Here's how the part is built. I have some questions about the finished solid (model axes, mm). Face numbers are marked on the shaded views. A direction names the side the tool comes from. Give positions to 0.01 mm unless a question says otherwise; leave off trailing zeros. Write each loop counter-clockwise with the first axis right and the second up, starting at its lowest first coordinate (ties: lowest second). Pieces come first, ordered by that corner, then holes. Notation, with made-up numbers: (12.25, 40) -> (71.25, 40) arc R26 cw to (71.25, 59) -> close; hole circle Ø7 at (69.5, 86.25). An arc over 180 degrees is marked (long way). Use one line per item in the form item = value.
```python
from build123d import *

# Parameters (mm, degrees)
SALIENTE_EXTRUIR2_DEPTH      = 2.5
SALIENTE_EXTRUIR2_DEPTH_BACK = 2.5
CROQUIS2_R                   = 8
CROQUIS2_R_2                 = 2.5
REDONDEO1_R                  = 0.5
REDONDEO2_R                  = 0.1
CROQUIS3_R                   = 7
CROQUIS3_R_2                 = 4
CORTAR_EXTRUIR1_DEPTH        = 0.1
CORTAR_EXTRUIR2_START        = -0.1
CROQUIS4_R                   = 7
CROQUIS4_R_2                 = 4
CORTAR_EXTRUIR2_DEPTH        = 0.1


with BuildPart() as part:
    # Croquis2 → Saliente-Extruir2 (new, two sides: drawn at the far end of the back side and taken through both)
    with BuildSketch(Plane(origin=(0, 0, 0), x_dir=(0, 0, -1), z_dir=(1, 0, 0)).offset(-SALIENTE_EXTRUIR2_DEPTH_BACK)):
        Circle(CROQUIS2_R)
        Circle(CROQUIS2_R_2, mode=Mode.SUBTRACT)
    extrude(amount=SALIENTE_EXTRUIR2_DEPTH + SALIENTE_EXTRUIR2_DEPTH_BACK)

    # Redondeo1
    redondeo1_edges = [part.edges().sort_by_distance(p)[0] for p in [
        (-2.5, 0, 8),
        (2.5, 0, 8),
    ]]
    fillet(redondeo1_edges, radius=REDONDEO1_R)

    # Redondeo2
    redondeo2_edges = [part.edges().sort_by_distance(p)[0] for p in [
        (-2.5, 0, 2.5),
        (2.5, 0, 2.5),
    ]]
    fillet(redondeo2_edges, radius=REDONDEO2_R)

    # Croquis3 → Cortar-Extruir1 (cut)
    with BuildSketch(Plane.ZY.offset(2.5)):
        Circle(CROQUIS3_R)
        Circle(CROQUIS3_R_2, mode=Mode.SUBTRACT)
    extrude(amount=-CORTAR_EXTRUIR1_DEPTH, mode=Mode.SUBTRACT)

    # Croquis4 → Cortar-Extruir2 (cut)
    with BuildSketch(Plane(origin=(2.5, 0, 0), x_dir=(0, 0, -1), z_dir=(1, 0, 0)).offset(CORTAR_EXTRUIR2_START)):
        with Locations(Location((0, 0, 0), (0, 0, 180))):
            Circle(CROQUIS4_R)
        with Locations(Location((0, 0, 0), (0, 0, 180))):
            Circle(CROQUIS4_R_2, mode=Mode.SUBTRACT)
    extrude(amount=CORTAR_EXTRUIR2_DEPTH, mode=Mode.SUBTRACT)


solid = part.part
```
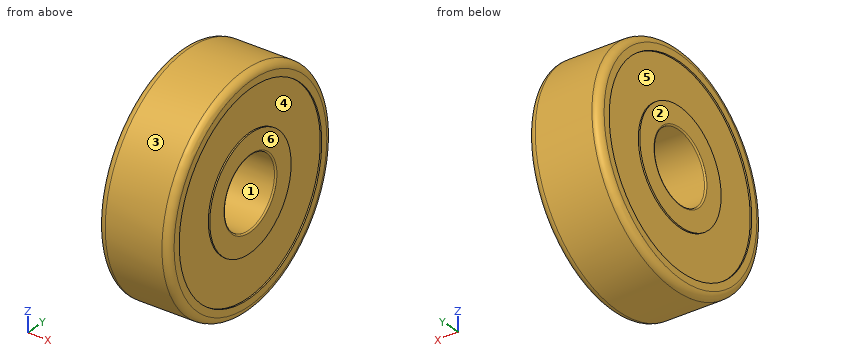
Q1. Will these pins go through, and if not, where does the flat tip stop? pin 1 Ø5 at (y, z) = (-1.5, -2) entering from -X; pin 2 Ø1 at (x, y) = (-2, 1) entering from +Z; pin 3 Ø1 at (y, z) = (-5.5, 0.5) entering from +X; pin 4 Ø1 at (x, z) = (1, 2.5) entering from +Y.
Result set:
pin_1 = -2.5
pin_2 = 7.98
pin_3 = 2.4
pin_4 = 7.75
Q2. Which directions (+Z, -Z, +X, -X, +Y, -Y) give clear straight access to the entire face, cutting with the end or side of a thin tool? Please do the marked faces 4, 5 and 6.
Result set:
face_4 = +X
face_5 = -X
face_6 = +Z, -Z, +X, +Y, -Y
Q3. If we mould it in two halves opening along Y, with no side actions, what happens to the marked faces 1, 2 and 3? For each: +Y half, -Y half, draft (parallel to the pull), parting line (faces both ways), or undercut.
Result set:
face_1 = undercut
face_2 = draft
face_3 = parting line
Q4. If I drill on line 1 along Y through (x, z) = (0.2, 0); line 2 along X through (y, z) = (-5, 0); line 3 along Z through (x, y) = (0.95, 1.75), over which ranges is the centre line in solid material (lowest first)? Write a range as from..to.
Result set:
line_1 = -8..-2.5, 2.5..8
line_2 = -2.4..2.4
line_3 = -7.81..-1.79, 1.79..7.81
Q5. I want a section at C-C, the plane x = -0.7. Write out the boundary of the cut face in (y, z), and give its area (3 significant figures).
Result set:
outline = circle Ø16 at (0, 0); hole circle Ø5 at (0, 0)
area = 181 mm2
